```python
from build123d import *

# Parameters (mm, degrees)
SKETCH1_R           = 2.6035
BOSS_EXTRUDE1_DEPTH = 152.4
SKETCH2_R           = 23.941884012
CUT_EXTRUDE1_DEPTH  = 247.396


with BuildPart() as part:
    # Sketch1 → Boss-Extrude1 (new, symmetric)
    with BuildSketch(Plane.XY):
        with BuildLine():
            Line((-7.179650497, -8.645192506), (-3.952270251, -5.423690499))
            ThreePointArc((-3.952270251, -5.423690499), (-2.922936451, -4.736929036), (-1.709253557, -4.4958))
            Line((-1.709253557, -4.4958), (1.709253557, -4.4958))
            ThreePointArc((1.709253557, -4.4958), (2.922936451, -4.736929036), (3.952270251, -5.423690499))
            Line((3.952270251, -5.423690499), (7.179650497, -8.645192506))
            ThreePointArc((7.179650497, -8.645192506), (7.41473083, -9.822813117), (6.416408329, -10.4902))
            Line((6.416408329, -10.4902), (4.287512407, -10.4902))
            ThreePointArc((4.287512407, -10.4902), (3.54574862, -10.79744862), (3.2385, -11.539212407))
            Line((3.2385, -11.539212407), (3.2385, -11.650987593))
            ThreePointArc((3.2385, -11.650987593), (3.54574862, -12.39275138), (4.287512407, -12.7))
            Line((4.287512407, -12.7), (5.317126718, -12.7))
            ThreePointArc((5.317126718, -12.7), (5.825126718, -12.192), (6.333126718, -12.7))
            Line((6.333126718, -12.7), (9.550443118, -12.7))
            ThreePointArc((9.550443118, -12.7), (10.058366869, -12.192000006), (10.566443095, -12.699847501))
            ThreePointArc((10.566443095, -12.699847501), (12.082537762, -12.08250727), (12.699846982, -10.566399977))
            ThreePointArc((12.699846982, -10.566399977), (12.192000006, -10.058323491), (12.7, -9.5504))
            Line((12.7, -9.5504), (12.7, -6.3330836))
            ThreePointArc((12.7, -6.3330836), (12.192, -5.8250836), (12.7, -5.3170836))
            Line((12.7, -5.3170836), (12.7, -4.287469289))
            ThreePointArc((12.7, -4.287469289), (12.39275138, -3.545705502), (11.650987593, -3.238456882))
            Line((11.650987593, -3.238456882), (11.539212407, -3.238456882))
            ThreePointArc((11.539212407, -3.238456882), (10.79744862, -3.545705502), (10.4902, -4.287469289))
            Line((10.4902, -4.287469289), (10.4902, -6.402089023))
            ThreePointArc((10.4902, -6.402089023), (9.856505071, -7.351067942), (8.737131347, -7.129408934))
            Line((8.737131347, -7.129408934), (5.441005833, -3.840816462))
            ThreePointArc((5.441005833, -3.840816462), (4.750877967, -2.809883091), (4.5085, -1.593185507))
            Line((4.5085, -1.593185507), (4.5085, 1.593185507))
            ThreePointArc((4.5085, 1.593185507), (4.750877967, 2.809883091), (5.441005833, 3.840816462))
            Line((5.441005833, 3.840816462), (8.737131347, 7.129408934))
            ThreePointArc((8.737131347, 7.129408934), (9.856505071, 7.351067942), (10.4902, 6.402089023))
            Line((10.4902, 6.402089023), (10.4902, 4.287469289))
            ThreePointArc((10.4902, 4.287469289), (10.79744862, 3.545705502), (11.539212407, 3.238456882))
            Line((11.539212407, 3.238456882), (11.650987593, 3.238456882))
            ThreePointArc((11.650987593, 3.238456882), (12.39275138, 3.545705502), (12.7, 4.287469289))
            Line((12.7, 4.287469289), (12.7, 5.3170836))
            ThreePointArc((12.7, 5.3170836), (12.192, 5.8250836), (12.7, 6.3330836))
            Line((12.7, 6.3330836), (12.7, 9.5504))
            ThreePointArc((12.7, 9.5504), (12.192000006, 10.058323491), (12.699846982, 10.566399977))
            ThreePointArc((12.699846982, 10.566399977), (12.082537762, 12.08250727), (10.566443095, 12.699847501))
            ThreePointArc((10.566443095, 12.699847501), (10.058366869, 12.192000006), (9.550443118, 12.7))
            Line((9.550443118, 12.7), (6.333126718, 12.7))
            ThreePointArc((6.333126718, 12.7), (5.825126718, 12.192), (5.317126718, 12.7))
            Line((5.317126718, 12.7), (4.287512407, 12.7))
            ThreePointArc((4.287512407, 12.7), (3.54574862, 12.39275138), (3.2385, 11.650987593))
            Line((3.2385, 11.650987593), (3.2385, 11.539212407))
            ThreePointArc((3.2385, 11.539212407), (3.54574862, 10.79744862), (4.287512407, 10.4902))
            Line((4.287512407, 10.4902), (6.476788598, 10.4902))
            ThreePointArc((6.476788598, 10.4902), (7.432222385, 9.85140422), (7.207036008, 8.724370562))
            Line((7.207036008, 8.724370562), (3.898272566, 5.423169045))
            ThreePointArc((3.898272566, 5.423169045), (2.869120213, 4.736787962), (1.655778399, 4.4958))
            Line((1.655778399, 4.4958), (-1.655778399, 4.4958))
            ThreePointArc((-1.655778399, 4.4958), (-2.869120213, 4.736787962), (-3.898272566, 5.423169045))
            Line((-3.898272566, 5.423169045), (-7.207036008, 8.724370562))
            ThreePointArc((-7.207036008, 8.724370562), (-7.432222385, 9.85140422), (-6.476788598, 10.4902))
            Line((-6.476788598, 10.4902), (-4.287512407, 10.4902))
            ThreePointArc((-4.287512407, 10.4902), (-3.54574862, 10.79744862), (-3.2385, 11.539212407))
            Line((-3.2385, 11.539212407), (-3.2385, 11.650987593))
            ThreePointArc((-3.2385, 11.650987593), (-3.54574862, 12.39275138), (-4.287512407, 12.7))
            Line((-4.287512407, 12.7), (-5.317126718, 12.7))
            ThreePointArc((-5.317126718, 12.7), (-5.825126718, 12.192), (-6.333126718, 12.7))
            Line((-6.333126718, 12.7), (-9.550443118, 12.7))
            ThreePointArc((-9.550443118, 12.7), (-10.058366869, 12.192000006), (-10.566443095, 12.699847501))
            ThreePointArc((-10.566443095, 12.699847501), (-12.082537762, 12.08250727), (-12.699846982, 10.566399977))
            ThreePointArc((-12.699846982, 10.566399977), (-12.192000006, 10.058323491), (-12.7, 9.5504))
            Line((-12.7, 9.5504), (-12.7, 6.3330836))
            ThreePointArc((-12.7, 6.3330836), (-12.192, 5.8250836), (-12.7, 5.3170836))
            Line((-12.7, 5.3170836), (-12.7, 4.287469289))
            ThreePointArc((-12.7, 4.287469289), (-12.39275138, 3.545705502), (-11.650987593, 3.238456882))
            Line((-11.650987593, 3.238456882), (-11.539212407, 3.238456882))
            ThreePointArc((-11.539212407, 3.238456882), (-10.79744862, 3.545705502), (-10.4902, 4.287469289))
            Line((-10.4902, 4.287469289), (-10.4902, 6.402089023))
            ThreePointArc((-10.4902, 6.402089023), (-9.856505071, 7.351067942), (-8.737131347, 7.129408934))
            Line((-8.737131347, 7.129408934), (-5.441005833, 3.840816462))
            ThreePointArc((-5.441005833, 3.840816462), (-4.750877967, 2.809883091), (-4.5085, 1.593185507))
            Line((-4.5085, 1.593185507), (-4.5085, -1.593185507))
            ThreePointArc((-4.5085, -1.593185507), (-4.750877967, -2.809883091), (-5.441005833, -3.840816462))
            Line((-5.441005833, -3.840816462), (-8.737131347, -7.129408934))
            ThreePointArc((-8.737131347, -7.129408934), (-9.856505071, -7.351067942), (-10.4902, -6.402089023))
            Line((-10.4902, -6.402089023), (-10.4902, -4.287469289))
            ThreePointArc((-10.4902, -4.287469289), (-10.79744862, -3.545705502), (-11.539212407, -3.238456882))
            Line((-11.539212407, -3.238456882), (-11.650987593, -3.238456882))
            ThreePointArc((-11.650987593, -3.238456882), (-12.39275138, -3.545705502), (-12.7, -4.287469289))
            Line((-12.7, -4.287469289), (-12.7, -5.3170836))
            ThreePointArc((-12.7, -5.3170836), (-12.192, -5.8250836), (-12.7, -6.3330836))
            Line((-12.7, -6.3330836), (-12.7, -9.5504))
            ThreePointArc((-12.7, -9.5504), (-12.192000006, -10.058323491), (-12.699846982, -10.566399977))
            ThreePointArc((-12.699846982, -10.566399977), (-12.082537762, -12.08250727), (-10.566443095, -12.699847501))
            ThreePointArc((-10.566443095, -12.699847501), (-10.058366869, -12.192000006), (-9.550443118, -12.7))
            Line((-9.550443118, -12.7), (-6.333126718, -12.7))
            ThreePointArc((-6.333126718, -12.7), (-5.825126718, -12.192), (-5.317126718, -12.7))
            Line((-5.317126718, -12.7), (-4.287512407, -12.7))
            ThreePointArc((-4.287512407, -12.7), (-3.54574862, -12.39275138), (-3.2385, -11.650987593))
            Line((-3.2385, -11.650987593), (-3.2385, -11.539212407))
            ThreePointArc((-3.2385, -11.539212407), (-3.54574862, -10.79744862), (-4.287512407, -10.4902))
            Line((-4.287512407, -10.4902), (-6.416408329, -10.4902))
            ThreePointArc((-6.416408329, -10.4902), (-7.41473083, -9.822813117), (-7.179650497, -8.645192506))
        make_face()
        with Locations(Location((0, 0, 0), (0, 0, 180))):
            Circle(SKETCH1_R, mode=Mode.SUBTRACT)
    extrude(amount=BOSS_EXTRUDE1_DEPTH, both=True)

    # Sketch2 → Cut-Extrude1 (cut)
    with BuildSketch(Plane.XY.offset(152.4)):
        Circle(SKETCH2_R)
    extrude(amount=-CUT_EXTRUDE1_DEPTH, mode=Mode.SUBTRACT)


solid = part.part
```
CAD build for the part. Positions are in the model's coordinates, mm. A direction names the side the tool comes from. Coordinates: 2 decimals unless noted, no trailing zeros. Loops run counter-clockwise (first coordinate to the right, second up) from the corner with the lowest first, then second, coordinate; pieces in that order, holes last. Notation, with made-up numbers: (14, 74.25) - (37, 74.25) arc R12 ccw to (37, 95.25) - close; hole circle Ø11 at (-10.75, 1). An arc over 180 degrees is marked (long way). Use CSV: the item, a comma, the result in double quotes. Start each with the question number.
Q1. Two-plate mould, pull along Y, no slides. Class faces 4 (the cylindrical face through (12.192, -10.069, -123.296)), 5 (the cylindrical face through (3.538, -12.385, -123.296)), 6 (the flat face through (-12.7, -8, -123)): +Y half, -Y half, draft (parallel to the pull), parting line (faces both ways), or undercut.
Q2. Cut at B-B, the plane x = 0. List the corners of the cut face in (y, z).
Q3. Probe probe 1 along Y at (x, z) = (0, -132.5); probe 2 along X at (y, z) = (-5.25, -103.5); probe 3 along Y at (x, z) = (2, -105.5). List the from-to ranges inside material, lowest first. Write a range as from..to.
Q4. Cut at A-A, the plane y = 0. List the corners of the cut face in (x, z), then the cut area to 3 significant figures.
Q5. Drop flat-ended pins along their axis: P1, Ø1, axis at y = 0, z = -119, coming from the -X side; P2, Ø5, axis at x = -4, z = -137.5, coming from the -Y side; P3, Ø1, axis at y = 0, z = -119.5, coming from the +X side; P4, Ø1.5, axis at x = 3, z = -101, coming from the +Y side. Give the stop position or say it passes through.
Q6. 3-axis set-ups, long thin cutter, end or side, ignore diameter. For faces 1 (the cylindrical face through (-3.538, 12.385, -123.296)), 2 (the flat face through (-12.7, -5, -123)), 3 (the flat face through (10.49, 5, -123)): which of +Z, -Z, +X, -X, +Y, -Y reach the whole face in a straight line?
Here are the results:
1,face 4,"undercut"
1,face 5,"-Y half"
1,face 6,"draft"
2,outline,"(-4.5, -152.4) - (-2.6, -152.4) - (-2.6, -95) - (-4.5, -95) - close; (2.6, -152.4) - (4.5, -152.4) - (4.5, -95) - (2.6, -95) - close"
3,probe 1,"-4.5..-2.6, 2.6..4.5"
3,probe 2,"-12.7..-10.49, -6.85..-3.76, 3.76..6.85, 10.49..12.7"
3,probe 3,"-4.51..-1.67, 1.67..4.51"
4,outline,"(-4.51, -152.4) - (-2.6, -152.4) - (-2.6, -95) - (-4.51, -95) - close; (2.6, -152.4) - (4.51, -152.4) - (4.51, -95) - (2.6, -95) - close"
4,area,"219 mm2"
5,P1,"x = -4.51"
5,P2,"y = -12.7"
5,P3,"x = 4.51"
5,P4,"y = 12.55"
6,face 1,"+Z, -Z, +Y"
6,face 2,"+Z, -Z, -X, +Y, -Y"
6,face 3,"+Z, -Z"
